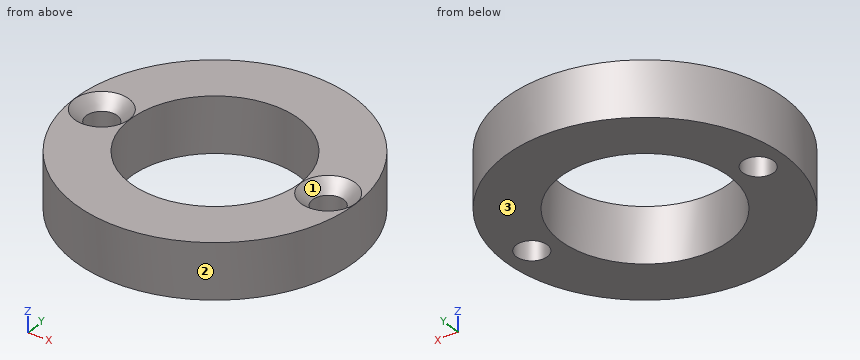
from build123d import *

# Parameters (mm, degrees)
SKETCH_R     = 20.25
SKETCH_R_2   = 12.25
SKETCH_R_3   = 2.25
PAD_DEPTH    = 8
CHAMFER_SIZE = 1.7


with BuildPart() as part:
    # Sketch → Pad (new body)
    with BuildSketch(Plane.XY):
        Circle(SKETCH_R)
        Circle(SKETCH_R_2, mode=Mode.SUBTRACT)
        with Locations((16.25, 0)):
            Circle(SKETCH_R_3, mode=Mode.SUBTRACT)
        with Locations((-16.25, 0)):
            Circle(SKETCH_R_3, mode=Mode.SUBTRACT)
    extrude(amount=PAD_DEPTH)

    # Chamfer
    chamfer_edges = [part.edges().sort_by_distance(p)[0] for p in [
        (14, 0, 8),
        (-18.5, 0, 8),
    ]]
    chamfer(chamfer_edges, length=CHAMFER_SIZE)


solid = part.part
CAD build for the part. Positions are in the model's coordinates, mm. Face numbers are marked on the shaded views. Round coordinates to 2 decimals unless told otherwise and drop trailing zeros. Write each loop counter-clockwise with the first axis right and the second up, starting at its lowest first coordinate (ties: lowest second). Pieces come first, ordered by that corner, then holes. Notation, with made-up numbers: M -18,85.5 L 31,85.5 A34 ccw 31,124.5 Z; hole C 1.25,-21 d10. An arc over 180 degrees is marked long. Use a Markdown table: item, result. Add a question column.
1. Flat gauge pins, fed straight in: P1, Ø4, axis at x = -16.25, y = 0, coming from the -Z side; P2, Ø3, axis at y = -6, z = 1, coming from the +X side; P3, Ø1.5, axis at y = -11, z = 2, coming from the -X side; P4, Ø2, axis at x = 10, z = 1.5, coming from the +Y side. Where does each tip first touch, or does it go through?
2. Slice it at A-A on y = 0. Give the cut face in (x, z).
3. Slice it at B-B on x = 0. Give the cut face in (y, z).
4. Drill centre lines: probe 1 along X at (y, z) = (-1.5, 1); probe 2 along Y at (x, z) = (0, 5.5); probe 3 along X at (y, z) = (-3, 2). Where is each one in solid material? Low to high.
5. Pull direction X, two halves, no side cores. Call the marked faces 1, 2 and 3: released by +X, released by -X, zero draft, split by the parting line, or undercut.
6. Slice it at D-D on z = 3.75. Give the cut face in (x, y), then the cut area to 3 significant figures.
7. Slice it at C-C on y = 10.5. Give the cut face in (x, z), then the cut area to 3 significant figures.
Reply:
| question | item | result |
|---|---|---|
| 1 | P1 | passes through |
| 1 | P2 | stops at x = 19.74 |
| 1 | P3 | stops at x = -17.46 |
| 1 | P4 | stops at y = 18.14 |
| 2 | outline | M -20.25,0 L -18.5,0 L -18.5,6.3 L -20.2,8 L -20.25,8 Z; M -14,0 L -12.25,0 L -12.25,8 L -12.3,8 L -14,6.3 Z; M 12.25,0 L 14,0 L 14,6.3 L 12.3,8 L 12.25,8 Z; M 18.5,0 L 20.25,0 L 20.25,8 L 20.2,8 L 18.5,6.3 Z |
| 3 | outline | M -20.25,0 L -12.25,0 L -12.25,8 L -20.25,8 Z; M 12.25,0 L 20.25,0 L 20.25,8 L 12.25,8 Z |
| 4 | probe 1 | x = -20.19 to -17.93, -14.57 to -12.16, 12.16 to 14.57, 17.93 to 20.19 |
| 4 | probe 2 | y = -20.25 to -12.25, 12.25 to 20.25 |
| 4 | probe 3 | x = -20.03 to -11.88, 11.88 to 20.03 |
| 5 | face 1 | undercut |
| 5 | face 2 | split by the parting line |
| 5 | face 3 | zero draft |
| 6 | outline | C 0,0 d40.5; hole C -16.25,0 d4.5; hole C 0,0 d24.5; hole C 16.25,0 d4.5 |
| 6 | area | 785 mm^2 |
| 7 | outline | M -17.32,0 L -6.31,0 L -6.31,8 L -17.32,8 Z; M 6.31,0 L 17.32,0 L 17.32,8 L 6.31,8 Z |
| 7 | area | 176 mm^2 |
